Answer from the drawing. Dimensions are ordinates in mm from the lowest x, y and z of the part. Round coordinates to 2 decimals unless told otherwise and drop trailing zeros. Loops run counter-clockwise (first coordinate to the right, second up) from the corner with the lowest first, then second, coordinate; pieces in that order, holes last.
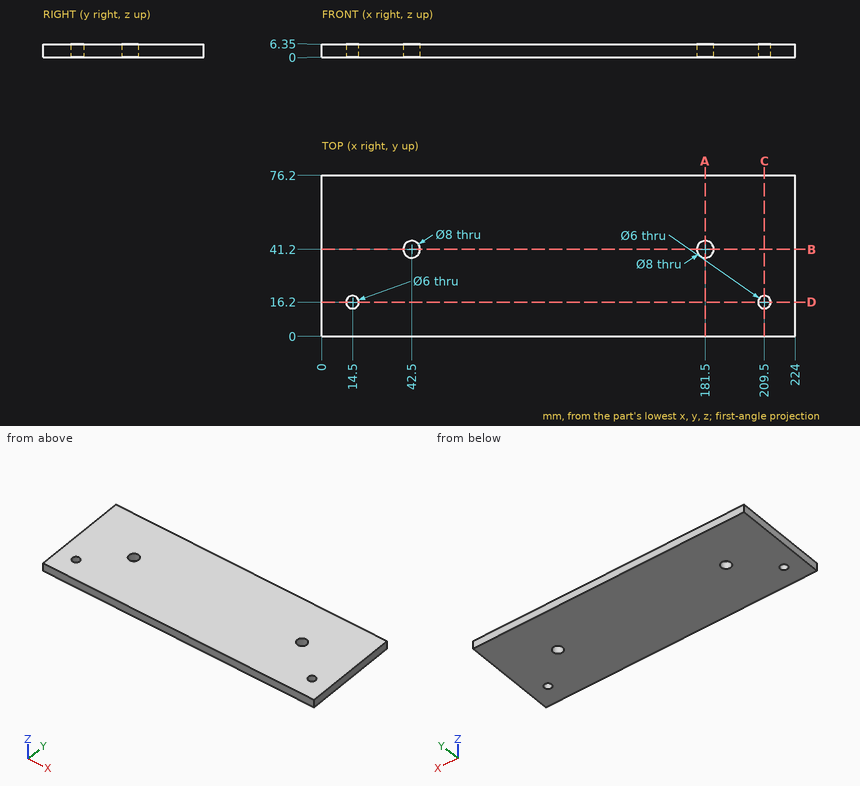
1. Find section D-D (y = 16.2). Write down the section's boundary in (x, z).
Answer key:
outline: (0, 0) - (11.5, 0) - (11.5, 6.35) - (0, 6.35) - close; (17.5, 0) - (206.5, 0) - (206.5, 6.35) - (17.5, 6.35) - close; (212.5, 0) - (224, 0) - (224, 6.35) - (212.5, 6.35) - close
2. Find section B-B (y = 41.2). Write down the section's boundary in (x, z), then the cut area to 3 significant figures.
Answer key:
outline: (0, 0) - (38.5, 0) - (38.5, 6.35) - (0, 6.35) - close; (46.5, 0) - (177.5, 0) - (177.5, 6.35) - (46.5, 6.35) - close; (185.5, 0) - (224, 0) - (224, 6.35) - (185.5, 6.35) - close
area: 1,320 mm2
3. Find section A-A (x = 181.5). Write down the section's boundary in (y, z), then the cut area to 3 significant figures.
Answer key:
outline: (0, 0) - (37.2, 0) - (37.2, 6.35) - (0, 6.35) - close; (45.2, 0) - (76.2, 0) - (76.2, 6.35) - (45.2, 6.35) - close
area: 433 mm2
4. Consider probe 1 along Y at (x, z) = (181.5, 3.75); probe 2 along Y at (x, z) = (209.5, 1.5). Determine where each line is inside the solid, lowest interval first.
Answer key:
probe 1: y = 0 to 37.2, 45.2 to 76.2
probe 2: y = 0 to 13.2, 19.2 to 76.2
5. Find section C-C (x = 209.5). Write down the section's boundary in (y, z).
Answer key:
outline: (0, 0) - (13.2, 0) - (13.2, 6.35) - (0, 6.35) - close; (19.2, 0) - (76.2, 0) - (76.2, 6.35) - (19.2, 6.35) - close
6. Given pin 1 (5 mm diameter, centred on x = 181.5, y = 41.2, fed in from -Z), flat-ended and moving along its own axis, determine where the tip first touches the part or whether it passes through.
Answer key:
pin 1: passes through
